Could you check a few things on this model? Use its own coordinates, in mm. A direction names the side the tool comes from. Coordinates: 2 decimals unless noted, no trailing zeros. Order: outer loops, then holes, each group sorted by start corner. A loop starts at its lowest first (then second) coordinate and runs counter-clockwise, first axis right, second up. Notation, with made-up numbers: (88.5, 14.5) -> (104.5, 14.5) arc R20 cw to (104.5, 53.5) -> close; hole circle Ø2 at (1, -12). An arc over 180 degrees is marked (long way). Return JSON: item names as keys, results as strings. Group by question number.
from build123d import *

# Parameters (mm, degrees)
SKIZZE1_R                       = 3.5
AUFSATZ_LINEAR_AUSTRAGEN1_DEPTH = 5.5
SKIZZE2_R                       = 5.5
AUFSATZ_LINEAR_AUSTRAGEN2_DEPTH = 2
SKIZZE3_R                       = 2
SCHNITT_LINEAR_AUSTRAGEN1_DEPTH = 0.5
VERRUNDUNG1_R                   = 2


with BuildPart() as part:
    # Skizze1 → Aufsatz-Linear austragen1 (new body)
    with BuildSketch(Plane(origin=(0, 0, 0), x_dir=(1, 0, 0), z_dir=(0, 1, 0))):
        Circle(SKIZZE1_R)
    extrude(amount=AUFSATZ_LINEAR_AUSTRAGEN1_DEPTH)

    # Skizze2 → Aufsatz-Linear austragen2 (add)
    with BuildSketch(Plane.XZ):
        Circle(SKIZZE2_R)
    extrude(amount=AUFSATZ_LINEAR_AUSTRAGEN2_DEPTH)

    # Skizze3 → Schnitt-Linear austragen1 (cut)
    with BuildSketch(Plane.XZ.offset(2)):
        Circle(SKIZZE3_R)
    extrude(amount=-SCHNITT_LINEAR_AUSTRAGEN1_DEPTH, mode=Mode.SUBTRACT)

    # Verrundung1
    verrundung1_edges = [part.edges().sort_by_distance(p)[0] for p in [
        (-3.5, 5.5, 0),
    ]]
    fillet(verrundung1_edges, radius=VERRUNDUNG1_R)


solid = part.part
Q1. I want a section at A-A on y = 2. Please give me the cut outline in (x, z), and give its area (3 significant figures).
Q2. On a 3-axis mill with a long thin cutter (end or side, diameter ignored), from which of +Z, -Z, +X, -X, +Y, -Y can I reach the whole of each face in a straight line? I mean faces 5 (the flat face through (4, 0, 0)), 6 (the flat face through (0, 5.5, 0)). Say none if no direction works.
Q3. I want a section at B-B on z = -3.75. Please give me the cut outline in (x, y), and give its area (3 significant figures).
Q4. I need wall thicknesses on line 1 along Z through (x, y) = (0, -1.7); line 2 along Y through (x, z) = (0, 1.5); line 3 along Y through (x, z) = (0.5, 4.75). Which ranges of each line are inside material? Lowest first, please. Write a range as from..to.
Q5. I want a section at C-C on x = 4.5. Please give me the cut outline in (y, z).
Q6. We'd pull the mould along Z, two halves only. Please class faces 1 (the flat face through (0, -1.5, 0)), 2 (the flat face through (-0.1, -2, -2.4)), 3 (the cylindrical face through (-1.19, -0.99, -5.37)), 4 (the cylindrical face through (-0.434, -1.754, -1.952)): pulls with the +Z half, pulls with the -Z half, needs draft (parallel to the pull), parting line crosses it, or undercut.
Q7. I'm going to push flat-ended pins straight in: pin 1 Ø3 at (x, z) = (-4, 4) entering from -Y; pin 2 Ø1.2 at (x, z) = (-1, 0.5) entering from -Y; pin 3 Ø1.5 at (x, z) = (-0.5, 2.5) entering from +Y. Where does each tip first touch, or does it pass through?
Response values:
{
 "1": {"outline": "circle Ø7 at (0, 0)", "area": "38.5 mm²"},
 "2": {"face 5": "+Y", "face 6": "+Z, -Z, +X, -X, +Y"},
 "3": {"outline": "(-4.02, -2) -> (4.02, -2) -> (4.02, 0) -> (-4.02, 0) -> close", "area": "16.1 mm²"},
 "4": {"line 1": "z = -5.5..-2, 2..5.5", "line 2": "y = -1.5..5.5", "line 3": "y = -2..0"},
 "5": {"outline": "(-2, -3.16) -> (0, -3.16) -> (0, 3.16) -> (-2, 3.16) -> close"},
 "6": {"face 1": "undercut", "face 2": "needs draft", "face 3": "parting line crosses it", "face 4": "undercut"},
 "7": {"pin 1": "stops at y = -2", "pin 2": "stops at y = -1.5", "pin 3": "stops at y = 5.48"}
}
